```python
from build123d import *

# Parameters (mm, degrees)
F1_DEPTH = 40.132
F3_DEPTH = 49.784


with BuildPart() as f1:
    # F0 (on Top) → F1 (new body)
    with BuildSketch(Plane.XY):
        with BuildLine():
            Line((-53.505063, -34.70511), (53.505063, -34.70511))
            Line((53.505063, -34.70511), (53.505063, -20.677222))
            ThreePointArc((53.505063, -20.677222), (32.827841, 0), (53.505063, 20.677222))
            Line((53.505063, 20.677222), (53.505063, 34.70511))
            Line((53.505063, 34.70511), (-53.505063, 34.70511))
            Line((-53.505063, 34.70511), (-53.505063, -34.70511))
        make_face()
    extrude(amount=F1_DEPTH)

    # F2 (on face) → F3 (cut)
    with BuildSketch(Plane(origin=(-53.505063, 0, 0), x_dir=(0, -1, 0), z_dir=(-1, 0, 0))):
        with BuildLine():
            Line((34.70511, 40.132), (5.878478, 40.132))
            ThreePointArc((5.878478, 40.132), (14.321603, 19.748493), (34.70511, 11.305368))
            Line((34.70511, 11.305368), (34.70511, 40.132))
        make_face()
        with BuildLine():
            ThreePointArc((34.70511, 11.305368), (55.088617, 19.748493), (63.531742, 40.132))
            ThreePointArc((63.531742, 40.132), (34.70511, 68.958632), (5.878478, 40.132))
            Line((5.878478, 40.132), (34.70511, 40.132))
            Line((34.70511, 40.132), (34.70511, 11.305368))
        make_face()
    extrude(amount=-F3_DEPTH, mode=Mode.SUBTRACT)


solid = f1.part
```
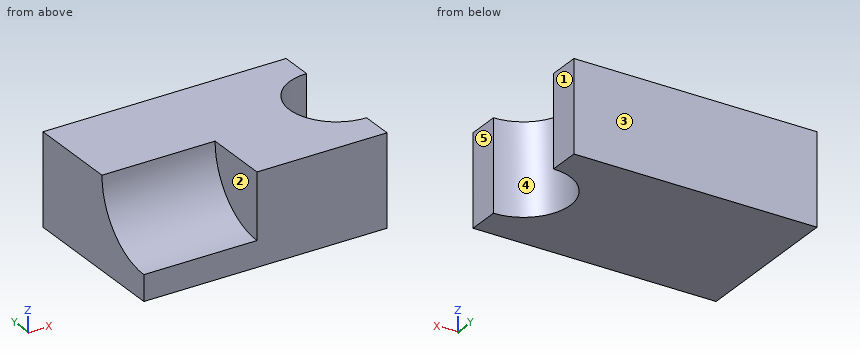
Source: CAD feature listing. Evaluate the final solid. Frame: model axes, mm. Face numbers are marked on the shaded views. A direction names the side the tool comes from. Coordinates: 2 decimals unless noted, no trailing zeros. Loops run counter-clockwise (first coordinate to the right, second up) from the corner with the lowest first, then second, coordinate; pieces in that order, holes last. Notation, with made-up numbers: M 82.5,14 L 101.5,14 A27 cw 101.5,39 Z; hole C 60.5,-7 d6. An arc over 180 degrees is marked long. Use a Markdown table: item, result. Add a question column.
Q1. First-contact query: pin 1 (8 mm diameter, centred on x = -41.5, y = -24, fed in from +Z); pin 2 (23 mm diameter, centred on y = -21, z = 27.5, fed in from -X). Flat tips, straight axial feed; report the tip coordinate or a pass-through.
Q2. Section query C-C, the plane x = -15. Return loops of the section in (y, z).
Q3. Section query A-A, the plane x = 45. Return loops of the section in (y, z).
Q4. Draft query along Y for the marked faces 3, 4 and 5. Return one class per face: pulls with the +Y half, pulls with the -Y half, needs draft (parallel to the pull), parting line crosses it, or undercut.
Q5. Material intervals for L1, parallel to Y at x = 49, z = 16; L2, parallel to Y at x = 41, z = 12; L3, parallel to X at y = 10.5, z = 30.5, sorted ascending.
Q6. Section query D-D, the plane y = 0. Return loops of the section in (x, z).
Q7. Access query for the marked faces 1 and 2. Directions: +Z, -Z, +X, -X, +Y, -Y. A direction counts if a zero-diameter tool reaches every point of the face in a straight line with its end or side. Return the directions, or none.
Q8. Section query B-B, the plane z = 9.5. Return loops of the section in (x, y), and give its area (3 significant figures).
Result:
| question | item | result |
|---|---|---|
| 1 | pin 1 | stops at z = 15.34 |
| 1 | pin 2 | stops at x = -53.51 |
| 2 | outline | M -34.71,0 L 34.71,0 L 34.71,40.13 L -5.88,40.13 A28.83 cw -34.71,11.31 Z |
| 3 | outline | M -34.71,0 L -18.85,0 L -18.85,40.13 L -34.71,40.13 Z; M 18.85,0 L 34.71,0 L 34.71,40.13 L 18.85,40.13 Z |
| 4 | face 3 | pulls with the +Y half |
| 4 | face 4 | undercut |
| 4 | face 5 | needs draft |
| 5 | L1 | y = -34.71 to -20.18, 20.18 to 34.71 |
| 5 | L2 | y = -34.71 to -16.47, 16.47 to 34.71 |
| 5 | L3 | x = -53.51 to 35.69 |
| 6 | outline | M -53.51,0 L 32.83,0 L 32.83,40.13 L -53.51,40.13 Z |
| 7 | face 1 | +Z, -Z, +X, +Y, -Y |
| 7 | face 2 | +Z, -X, -Y |
| 8 | outline | M -53.51,-34.71 L 53.51,-34.71 L 53.51,-20.68 A20.68 cw 53.51,20.68 L 53.51,34.71 L -53.51,34.71 Z |
| 8 | area | 6,760 mm2 |
